Can you work these out from the model? Positions are in its coordinate system, mm. A direction names the side the tool comes from. Give positions to 0.01 mm unless a question says otherwise; leave off trailing zeros. Loops run counter-clockwise (first coordinate to the right, second up) from the corner with the lowest first, then second, coordinate; pieces in that order, holes last. Notation, with made-up numbers: (-4.5, -9.5) -> (0.5, -9.5) arc R36 cw to (0.5, 28.5) -> close; hole circle Ø5 at (53.25, -6.5). An arc over 180 degrees is marked (long way). One line per question, with ' | ' between items.
from build123d import *

# Parameters (mm, degrees)
F0_R     = 12.5
F0_R_2   = 10.5
F1_DEPTH = 9.3
F0_R_3   = 1.5
F0_R_4   = 2.2
F2_DEPTH = 6
F3_R     = 1.5
F4_DEPTH = 3


with BuildPart() as f1:
    # F0 (on Front) → F1 (new body)
    with BuildSketch(Plane.XZ):
        Circle(F0_R)
        Circle(F0_R_2, mode=Mode.SUBTRACT)
    extrude(amount=F1_DEPTH)

    # F0 (on Front) → F2 (join)
    with BuildSketch(Plane.XZ):
        Circle(F0_R_2)
        with Locations((-6.3, 0)):
            Circle(F0_R_3, mode=Mode.SUBTRACT)
        Circle(F0_R_4, mode=Mode.SUBTRACT)
        with Locations((6.3, 0)):
            Circle(F0_R_3, mode=Mode.SUBTRACT)
    extrude(amount=F2_DEPTH)

    # F3 (on face) → F4 (cut)
    with BuildSketch(Plane(origin=(0, 0, 0), x_dir=(-1, 0, 0), z_dir=(0, 1, 0))):
        Polygon((-4.63207, -2.847532), (-3, 0.020704), (-4.66793, 2.868236), (-7.96793, 2.847532), (-9.6, -0.020704), (-7.93207, -2.868236), align=None)
        with Locations((-6.3, 0)):
            Circle(F3_R, mode=Mode.SUBTRACT)
        Polygon((7.93207, -2.868236), (9.6, -0.020704), (7.96793, 2.847532), (4.66793, 2.868236), (3, 0.020704), (4.63207, -2.847532), align=None)
        with Locations((6.3, 0)):
            Circle(F3_R, mode=Mode.SUBTRACT)
    extrude(amount=-F4_DEPTH, mode=Mode.SUBTRACT)


solid = f1.part
Q1. If we section it at C-C (z = -7): Write out the boundary of the cut face in (x, y), plus the area to 3 significant figures.
Entries:
outline: (-10.36, -9.3) -> (-7.83, -9.3) -> (-7.83, -6) -> (7.83, -6) -> (7.83, -9.3) -> (10.36, -9.3) -> (10.36, 0) -> (-10.36, 0) -> close | area: 141 mm²
Q2. If I drill on probe 1 along Z at (x, y) = (0, -3.1); probe 2 along Z at (x, y) = (0, -6.75); probe 3 along Y at (x, z) = (-8.25, 4.5), over which ranges is the centre line in solid material (lowest first)? Write a range as from..to.
Entries:
probe 1: -12.5..-2.2, 2.2..12.5 | probe 2: -12.5..-10.5, 10.5..12.5 | probe 3: -6..0
Q3. If we section it at B-B (y = -1.5): Write out the boundary of the cut face in (x, z), plus the area to 3 significant figures.
Entries:
outline: circle Ø25 at (0, 0); hole (-9.6, -0.02) -> (-7.93, -2.87) -> (-4.63, -2.85) -> (-3, 0.02) -> (-4.67, 2.87) -> (-7.97, 2.85) -> close; hole circle Ø4.4 at (0, 0); hole (3, 0.02) -> (4.63, -2.85) -> (7.93, -2.87) -> (9.6, -0.02) -> (7.97, 2.85) -> (4.67, 2.87) -> close | area: 419 mm²
Q4. If we section it at A-A (x = 0): Write out the boundary of the cut face in (y, z).
Entries:
outline: (-9.3, -12.5) -> (0, -12.5) -> (0, -2.2) -> (-6, -2.2) -> (-6, -10.5) -> (-9.3, -10.5) -> close; (-9.3, 10.5) -> (-6, 10.5) -> (-6, 2.2) -> (0, 2.2) -> (0, 12.5) -> (-9.3, 12.5) -> close
Q5. On a 3-axis mill with a long thin cutter (end or side, diameter ignored), from which of +Z, -Z, +X, -X, +Y, -Y can I reach the whole of each face in a straight line? I mean faces 1 (the face through (-4.87, -4.48, 0.45)), 2 (the face through (10, -7.6, 3.2)), 3 (the face through (-3.846, -1.479, 1.464)). Say none if no direction works.
Entries:
face 1: +Y, -Y | face 2: -Y | face 3: +Y
Q6. If we mould it in two halves opening along Z, with no side actions, what happens to faces 4 (the face through (11.923, -4.585, 3.755)), 5 (the face through (8.773, -1.479, 1.433)), 6 (the face through (2.6, 0, 0.2))? For each: pulls with the +Z half, pulls with the -Z half, needs draft (parallel to the pull), parting line crosses it, or undercut.
Entries:
face 4: parting line crosses it | face 5: undercut | face 6: needs draft
Q7. If we section it at D-D (x = 6.3): Write out the boundary of the cut face in (y, z).
Entries:
outline: (-9.3, -10.8) -> (0, -10.8) -> (0, -2.86) -> (-3, -2.86) -> (-3, -1.5) -> (-6, -1.5) -> (-6, -8.4) -> (-9.3, -8.4) -> close; (-9.3, 8.4) -> (-6, 8.4) -> (-6, 1.5) -> (-3, 1.5) -> (-3, 2.86) -> (0, 2.86) -> (0, 10.8) -> (-9.3, 10.8) -> close
Q8. For pin 1 Ø3 at (x, y) = (-5.5, -2) entering from -Z; pin 2 Ø1 at (x, y) = (2, -3.5) entering from -Z; pin 3 Ø1 at (x, y) = (-4, -5) entering from -Z; pin 4 Ø2.5 at (x, z) = (-6.3, 0) entering from +Y, each with a flat end and sliding along its axis, tell me the tip position at first contact or that it passes through.
Entries:
pin 1: z = -11.84 | pin 2: z = -12.41 | pin 3: z = -12 | pin 4: through
